Check sheet for the modelled part. Datum: model origin and axes. Units: mm. Face numbers are marked on the shaded views. Round coordinates to 2 decimals unless told otherwise and drop trailing zeros. Order: outer loops, then holes, each group sorted by start corner. A loop starts at its lowest first (then second) coordinate and runs counter-clockwise, first axis right, second up.
Q1. Scan lines: probe 1 along Z at (x, y) = (155, 14); probe 2 along X at (y, z) = (15, 440); probe 3 along X at (y, z) = (14, 400). Record each from-to range of solid material in increasing order.
Q2. Depth check by flat-ended pin: P1, Ø12, axis at y = -17, z = 160.5, coming from the +X side; P2, Ø16, axis at x = -10, z = 10, coming from the -Y side; P3, Ø12, axis at y = -4.5, z = 282, coming from the -X side. Enter the tip coordinate at first touch or a pass-through.
Q3. Cross-section at B-B on x = -10. Record the cut outline in (y, z), then the cut area to 3 significant figures.
Q4. Mould release check, pull along X, two halves, no side actions. Record for the marked faces 1 and 2: +X half, -X half, draft (parallel to the pull), parting line (faces both ways), or undercut.
Q5. Cross-section at D-D on x = 30. Record the cut outline in (y, z).
Q6. Cross-section at A-A on z = 10. Record the cut outline in (x, y), then the cut area to 3 significant figures.
Q7. Cross-section at C-C on z = 269.5. Record the cut outline in (x, y), then the cut area to 3 significant figures.
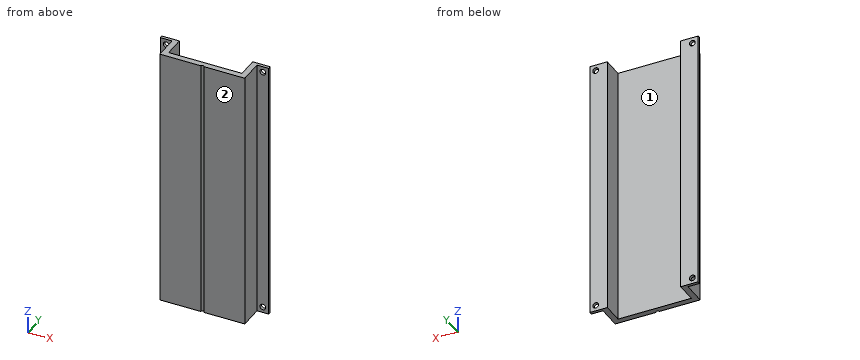
Autodesk Inventor part; units mm, degrees
ref_plane "YZ Plane" through (0, 0, 0) normal (1, 0, 0) x (0, 1, 0)
ref_plane "XZ Plane" through (0, 0, 0) normal (0, 1, 0) x (-1, 0, 0)
ref_plane "XY Plane" through (0, 0, 0) normal (0, 0, 1) x (1, 0, 0)
sketch "Sketch1" plane through (0, 0, 0) normal (0, 0, 1) x (1, 0, 0)
  line L0 (165.5, 18.25) -> (165.5, 13.25)
  line L1 (95.5, -27.5) -> (75.25, -27.5)
  arc A0 (75.25, -27.5) -> (70.25, -27.5) centre (72.75, -27.5) ccw
  line L2 (70.25, -27.5) -> (50, -27.5)
  line L3 (145.5, 0) -> (145.5, 13.25)
  line L4 (145.5, 13.25) -> (165.5, 13.25)
  line L5 (0, 13.25) -> (0, 0)
  line L6 (0, 13.25) -> (-20, 13.25)
  line L7 (-20, 13.25) -> (-20, 18.25)
  line L8 (-20, 18.25) -> (0, 18.25)
  line L9 (0, 18.25) -> (10, 18.25)
  line L10 (10, 18.25) -> (10, -17.5)
  line L11 (165.5, 18.25) -> (145.5, 18.25)
  line L12 (145.5, 18.25) -> (135.5, 18.25)
  line L13 (135.5, 18.25) -> (135.5, -17.5)
  line L14 (135.5, -17.5) -> (10, -17.5)
  line L15 (0, 0) -> (0, -27.5)
  line L16 (0, -27.5) -> (50, -27.5)
  line L17 (95.5, -27.5) -> (145.5, -27.5)
  line L18 (145.5, -27.5) -> (145.5, 0)
  point P0 (0, 0)
  dimension "d0" = 10
  dimension "d1" = 35.75
  dimension "d2" = 10
extrude "Extrusion1" add sketch "Sketch1" along normal blind 450
sketch "Sketch2" plane through (-20, 13.25, 0) normal (0, -1, 0) x (1, 0, 0)
  line L0 (30, 450) -> (0, 450)
  line L1 (20, 0) -> (20, 450)
  line L2 (0, 450) -> (20, 450)
  line L3 (20, 450) -> (20, 430)
  line L4 (20, 430) -> (0, 430)
  line L5 (0, 430) -> (0, 450)
  circle A0 centre (10, 440) radius 5
  line L6 (185.5, 0) -> (185.5, 450)
  line L7 (185.5, 450) -> (165.5, 450)
  line L8 (165.5, 450) -> (165.5, 430)
  line L9 (165.5, 430) -> (185.5, 430)
  line L10 (185.5, 430) -> (185.5, 450)
  line L11 (185.5, 0) -> (155.5, 0)
  line L12 (185.5, 0) -> (165.5, 0)
  line L13 (165.5, 0) -> (165.5, 20)
  line L14 (165.5, 20) -> (185.5, 20)
  line L15 (185.5, 20) -> (185.5, 0)
  line L16 (0, 0) -> (0, 450)
  line L17 (0, 0) -> (20, 0)
  line L18 (20, 0) -> (20, 20)
  line L19 (20, 20) -> (0, 20)
  line L20 (0, 20) -> (0, 0)
  circle A1 centre (175.5, 440) radius 5
  circle A2 centre (175.5, 10) radius 5
  circle A3 centre (10, 10) radius 5
  dimension "d5" = 20
  dimension "d6" = 10
  dimension "d7" = 20
  dimension "d8" = 20
  dimension "d9" = 20
  dimension "d10" = 20
  dimension "d11" = 20
  dimension "d12" = 20
  dimension "d13" = 10
  dimension "d14" = 10
  dimension "d15" = 10
extrude "Extrusion2" cut sketch "Sketch2" against normal blind 450 contours A0 | A1 | A2 | A3
properties part number "SoporteMaterial"
Results found:
1. probe 1: z = 0 to 5.03, 14.97 to 435.03, 444.97 to 450
1. probe 2: x = -20 to -15, -5 to 10, 135.5 to 150.5, 160.5 to 165.5
1. probe 3: x = -20 to 10, 135.5 to 165.5
2. P1: stops at x = 145.5
2. P2: stops at y = 13.25
2. P3: stops at x = 0
3. outline: (13.25, 0) - (18.25, 0) - (18.25, 5) - (13.25, 5) - close; (13.25, 15) - (18.25, 15) - (18.25, 435) - (13.25, 435) - close; (13.25, 445) - (18.25, 445) - (18.25, 450) - (13.25, 450) - close
3. area: 2,150 mm2
4. face 1: undercut
4. face 2: draft
5. outline: (-27.5, 0) - (-17.5, 0) - (-17.5, 450) - (-27.5, 450) - close
6. outline: (-20, 13.25) - (-15, 13.25) - (-15, 18.25) - (-20, 18.25) - close; (-5, 13.25) - (0, 13.25) - (0, -27.5) - (70.25, -27.5) arc R2.5 cw to (75.25, -27.5) - (145.5, -27.5) - (145.5, 13.25) - (150.5, 13.25) - (150.5, 18.25) - (135.5, 18.25) - (135.5, -17.5) - (10, -17.5) - (10, 18.25) - (-5, 18.25) - close; (160.5, 13.25) - (165.5, 13.25) - (165.5, 18.25) - (160.5, 18.25) - close
6. area: 2,260 mm2
7. outline: (-20, 13.25) - (0, 13.25) - (0, -27.5) - (70.25, -27.5) arc R2.5 cw to (75.25, -27.5) - (145.5, -27.5) - (145.5, 13.25) - (165.5, 13.25) - (165.5, 18.25) - (135.5, 18.25) - (135.5, -17.5) - (10, -17.5) - (10, 18.25) - (-20, 18.25) - close
7. area: 2,360 mm2
